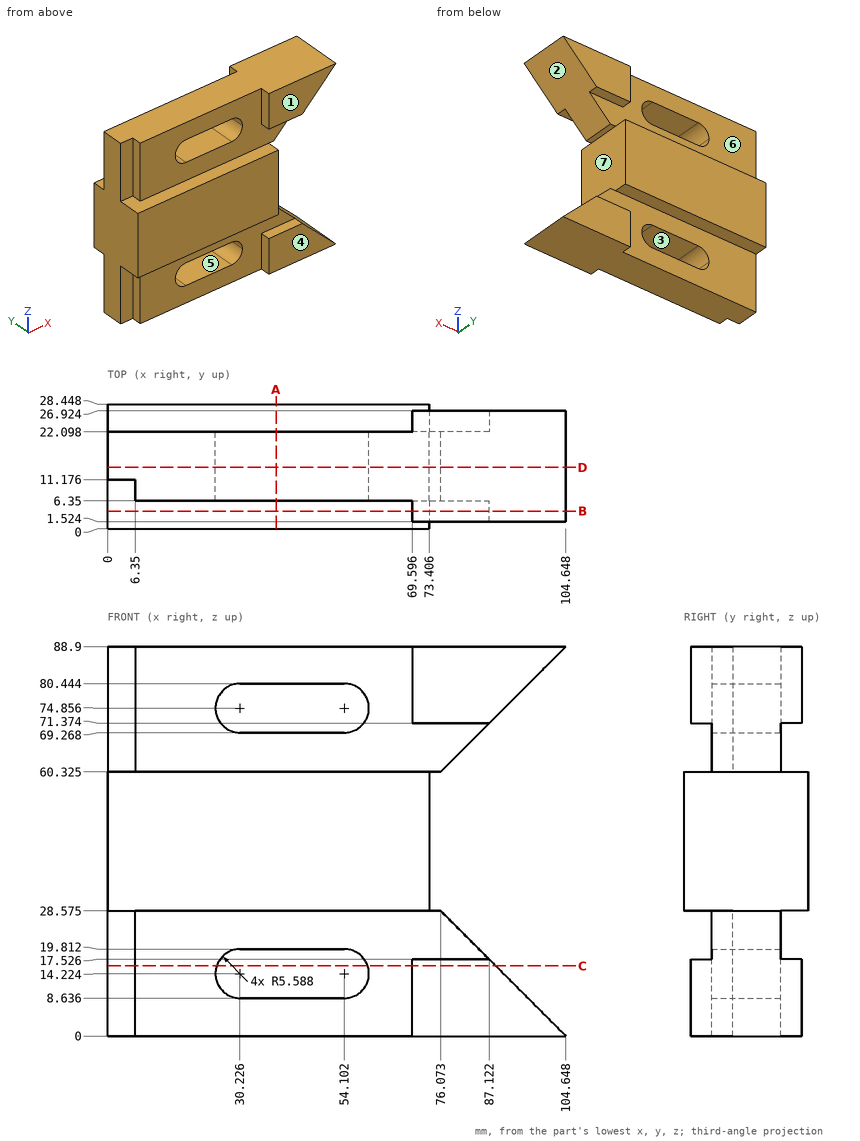
Design review of the part shown in the three views and the two pictorial views. Dimensions are in mm from the part's minimum x, y and z. A direction names the side the tool comes from. Round coordinates to 2 decimals unless told otherwise and drop trailing zeros. Loops run counter-clockwise (first coordinate to the right, second up) from the corner with the lowest first, then second, coordinate; pieces in that order, holes last. Notation, with made-up numbers: (-18.5, 22) - (8.5, 22) arc R14 ccw to (8.5, 31) - close; hole circle Ø9 at (24.5, 41.25). An arc over 180 degrees is marked (long way). One line per item, written item: value. Start each with the question number.
Item 1: Clearance check with flat-ended pins moving along their axes: pin 1 Ø1.5 at (y, z) = (19.5, 39) entering from +X; pin 2 Ø3 at (x, z) = (54, 66.5) entering from +Y; pin 3 Ø2.5 at (y, z) = (9, 9) entering from -X. State where each tip first meets the part, or that it passes through.
Item 2: For the marked faces 1, 2, 3 and 4, list the 3-axis set-ups (+Z, -Z, +X, -X, +Y, -Y) from which the entire face can be reached by the end or side of a thin tool; tool diameter is ignored.
Item 3: Take a section at B-B (y = 4). Give the boundary of the cut face in (x, z) (1 decimal), plus the area to 3 significant figures.
Item 4: Take a section at A-A (x = 38.5). State how many separate pieces and enclosed holes the cut face has, plus the area to 3 significant figures.
Item 5: The part is to be moulded in two halves that separate along X. For the marked faces 5, 6 and 7, say which applies: +X half, -X half, draft (parallel to the pull), parting line (faces both ways), or undercut.
Item 6: For L1, parallel to Y at x = 45, z = 83.5; L2, parallel to Z at x = 25, y = 2.25 (1 decimal); L3, parallel to X at y = 24.25, z = 46.5, list the stretches that pass through material, from the lowest coordinate up.
Item 7: Take a section at D-D (y = 14). Give the boundary of the cut face in (x, z) (1 decimal).
Item 8: Take a section at C-C (z = 16). Give the boundary of the cut face in (x, y), plus the area to 3 significant figures.
Answer below:
1. pin 1: stops at x = 73.41
1. pin 2: stops at y = 22.1
1. pin 3: stops at x = 6.35
2. face 1: +Z, +X, -X, -Y
2. face 2: +X, +Y, -Y
2. face 3: +Y, -Y
2. face 4: -Z, +X, -X, -Y
3. outline: (0, 28.6) - (73.4, 28.6) - (73.4, 60.3) - (0, 60.3) - close; (69.6, 0) - (104.6, 0) - (87.1, 17.5) - (69.6, 17.5) - close; (69.6, 71.4) - (87.1, 71.4) - (104.6, 88.9) - (69.6, 88.9) - close
3. area: 3,250 mm2
4. separate pieces: 3
4. enclosed holes: 0
4. area: 1,450 mm2
5. face 5: undercut
5. face 6: draft
5. face 7: +X half
6. L1: y = 6.35 to 22.1
6. L2: z = 28.6 to 60.3
6. L3: x = 0 to 73.41
7. outline: (0, 0) - (104.6, 0) - (76.1, 28.6) - (73.4, 28.6) - (73.4, 60.3) - (76.1, 60.3) - (104.6, 88.9) - (0, 88.9) - close; hole (30.2, 8.6) - (54.1, 8.6) arc R5.6 ccw to (54.1, 19.8) - (30.2, 19.8) arc R5.6 ccw to start; hole (30.2, 69.3) - (54.1, 69.3) arc R5.6 ccw to (54.1, 80.4) - (30.2, 80.4) arc R5.6 ccw to start
8. outline: (0, 11.18) - (6.35, 11.18) - (6.35, 6.35) - (24.93, 6.35) - (24.93, 22.1) - (0, 22.1) - close; (59.4, 6.35) - (69.6, 6.35) - (69.6, 1.52) - (88.65, 1.52) - (88.65, 26.92) - (69.6, 26.92) - (69.6, 22.1) - (59.4, 22.1) - close
8. area: 1,010 mm2
